Print and shaded views of the part. All mm, measured from the part's lowest x, y and z. Give positions to 0.01 mm unless a question says otherwise; leave off trailing zeros. Write each loop counter-clockwise with the first axis right and the second up, starting at its lowest first coordinate (ties: lowest second). Pieces come first, ordered by that corner, then holes. Notation, with made-up numbers: M 49,58 L 77,58 A20 cw 77,68 Z; hole C 68,-4 d5. An arc over 180 degrees is marked long. One line per question, with ' | ' between items. Start each with the question number.
1. Wall check: L1, parallel to X at y = 2.9, z = 0.65; L2, parallel to Y at x = 12, z = 0.55; L3, parallel to X at y = 2.7, z = 0.6. Give the ranges that are in metal, low to high.
2. Cut at B-B, the plane z = 0.45. Write the cut outline in (x, y).
3. Cut at A-A, the plane y = 2.5. Write the cut outline in (x, z), then the cut area to 3 significant figures.
4. Flat gauge pins, fed straight in: pin 1 (2 mm diameter, centred on x = 11, y = 3.5, fed in from -Z); pin 2 (2 mm diameter, centred on x = 12, y = 2.5, fed in from -Z). Where does each tip first touch, or does it go through?
5. Pull direction X, two halves, no side cores. Call the marked faces 1, 2, 3 and 4: released by +X, released by -X, zero draft, split by the parting line, or undercut.
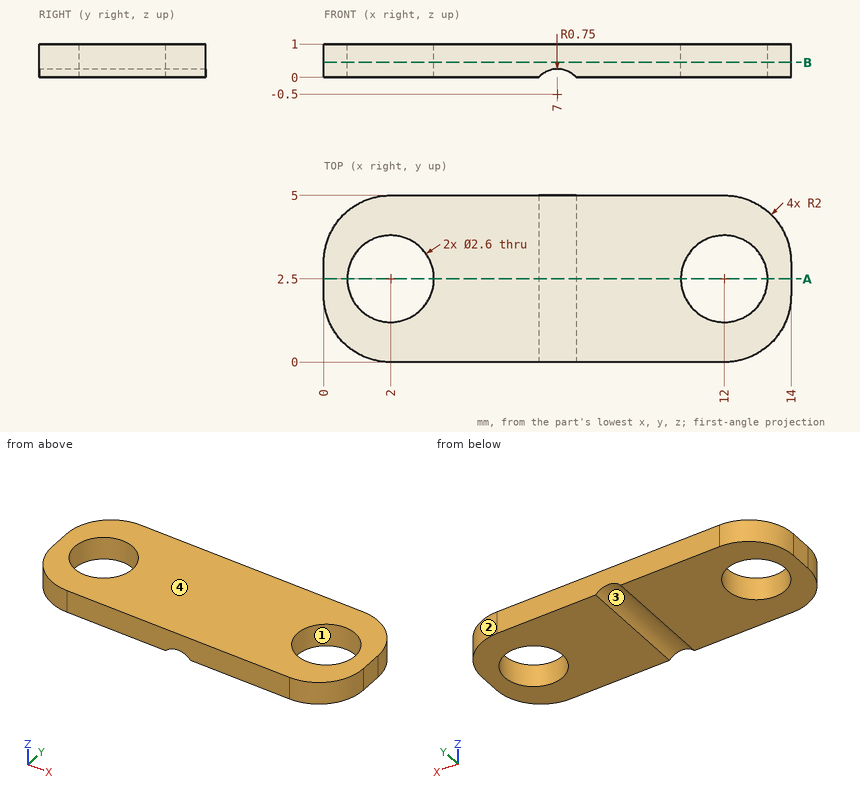
Here are the results:
1) L1: 0 to 0.76, 3.24 to 10.76, 13.24 to 14 | L2: 0 to 1.2, 3.8 to 5 | L3: 0 to 0.72, 3.28 to 10.72, 13.28 to 14
2) outline: M 0,2 A2 ccw 2,0 L 12,0 A2 ccw 14,2 L 14,3 A2 ccw 12,5 L 2,5 A2 ccw 0,3 Z; hole C 2,2.5 d2.6; hole C 12,2.5 d2.6
3) outline: M 0,0 L 0.7,0 L 0.7,1 L 0,1 Z; M 3.3,0 L 6.44,0 A0.75 cw 7.56,0 L 10.7,0 L 10.7,1 L 3.3,1 Z; M 13.3,0 L 14,0 L 14,1 L 13.3,1 Z | area: 8.61 mm^2
4) pin 1: z = 0 | pin 2: through
5) face 1: undercut | face 2: released by +X | face 3: undercut | face 4: zero draft
